Read the model definition and answer for the solid it produces. Units are mm, in the model's axes. Face numbers are marked on the shaded views. A direction names the side the tool comes from. Coordinates: 2 decimals unless noted, no trailing zeros. Order: outer loops, then holes, each group sorted by start corner. A loop starts at its lowest first (then second) coordinate and runs counter-clockwise, first axis right, second up. Notation, with made-up numbers: (-36, 19.25) -> (0, 19.25) arc R3 ccw to (0, 23.25) -> close; hole circle Ø8 at (-37.75, 85.25). An arc over 180 degrees is marked (long way). Answer as a JSON object with one key per item and string values. Group by question number.
1) Consider L1, parallel to Y at x = 0, z = 2.1; L2, parallel to Y at x = 0, z = 1.25; L3, parallel to Z at x = 3.5, y = 3.5. Determine where each line is inside the solid, lowest interval first.
2) A tool of negligible diameter and unlimited length cuts with its end or side. For the marked faces 1 and 2, from which of +Z, -Z, +X, -X, +Y, -Y can it reach the whole face along a straight path? Write none if from no direction.
3) Given pin 1 (8.5 mm diameter, centred on x = 3, y = 2, fed in from -Z); pin 2 (2 mm diameter, centred on y = 1.5, z = 8.5, fed in from -X); pin 3 (10 mm diameter, centred on x = 10, z = 10, fed in from +Y), each flat-ended and moving along its own axis, determine where each tip first touches the part or whether it passes through.
4) Determine the mould class of the marked faces 3, 4 and 5 for opening direction Y: released by +Y, released by -Y, zero draft, split by the parting line, or undercut.
5) Section A-A on x = 0 is taken. Determine the outline of the cut face in (y, z).
6) Section D-D on x = -15.5 is taken. Determine the outline of the cut face in (y, z).
7) Section C-C on z = 6 is taken. Determine the outline of the cut face in (x, y), and give its area (3 significant figures).
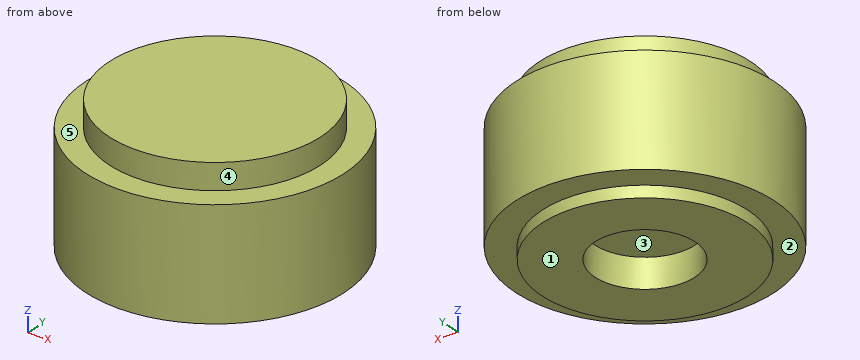
from build123d import *

# Parameters (mm, degrees)
F0_R     = 22
F0_R_2   = 17.5
F0_R_3   = 8.5
F1_DEPTH = 25
F2_DEPTH = 5
F3_DEPTH = 2
F4_R     = 22
F4_R_2   = 18
F5_DEPTH = 4.4


with BuildPart() as f1:
    # F0 (on Top) → F1 (new body)
    with BuildSketch(Plane.XY):
        Circle(F0_R)
        Circle(F0_R_2, mode=Mode.SUBTRACT)
        Circle(F0_R_2)
        Circle(F0_R_3, mode=Mode.SUBTRACT)
        Circle(F0_R_3)
    extrude(amount=F1_DEPTH)

    # F0 (on Top) → F2 (cut)
    with BuildSketch(Plane.XY):
        Circle(F0_R_3)
    extrude(amount=F2_DEPTH, mode=Mode.SUBTRACT)

    # F0 (on Top) → F3 (cut)
    with BuildSketch(Plane.XY):
        Circle(F0_R)
        Circle(F0_R_2, mode=Mode.SUBTRACT)
    extrude(amount=F3_DEPTH, mode=Mode.SUBTRACT)

    # F4 (on face) → F5 (cut)
    with BuildSketch(Plane.XY.offset(25)):
        Circle(F4_R)
        Circle(F4_R_2, mode=Mode.SUBTRACT)
    extrude(amount=-F5_DEPTH, mode=Mode.SUBTRACT)


solid = f1.part
Worked answers:
{
 "1": {"L1": "y = -22 to -8.5, 8.5 to 22", "L2": "y = -17.5 to -8.5, 8.5 to 17.5", "L3": "z = 5 to 25"},
 "2": {"face 1": "-Z, +X, -X, +Y, -Y", "face 2": "-Z"},
 "3": {"pin 1": "stops at z = 5", "pin 2": "stops at x = -21.99", "pin 3": "stops at y = 21.42"},
 "4": {"face 3": "undercut", "face 4": "split by the parting line", "face 5": "zero draft"},
 "5": {"outline": "(-22, 2) -> (-17.5, 2) -> (-17.5, 0) -> (-8.5, 0) -> (-8.5, 5) -> (8.5, 5) -> (8.5, 0) -> (17.5, 0) -> (17.5, 2) -> (22, 2) -> (22, 20.6) -> (18, 20.6) -> (18, 25) -> (-18, 25) -> (-18, 20.6) -> (-22, 20.6) -> close"},
 "6": {"outline": "(-15.61, 2) -> (-8.12, 2) -> (-8.12, 0) -> (8.12, 0) -> (8.12, 2) -> (15.61, 2) -> (15.61, 20.6) -> (9.15, 20.6) -> (9.15, 25) -> (-9.15, 25) -> (-9.15, 20.6) -> (-15.61, 20.6) -> close"},
 "7": {"outline": "circle Ø44 at (0, 0)", "area": "1,520 mm²"}
}
